```python
from build123d import *

# Parameters (mm, degrees)
CROQUIS1_W                 = 985
CROQUIS1_H                 = 100
SALIENTE_EXTRUIR1_DEPTH    = 12
CROQUIS2_R                 = 18.5
CORTAR_EXTRUIR1_DEPTH      = 1
CORTAR_EXTRUIR1_DEPTH_BACK = 13
CROQUIS3_R                 = 18.5
CORTAR_EXTRUIR2_DEPTH      = 13


with BuildPart() as part:
    # Croquis1 → Saliente-Extruir1 (new body)
    with BuildSketch(Plane.XY):
        with Locations((492.5, 50)):
            Rectangle(CROQUIS1_W, CROQUIS1_H)
    extrude(amount=SALIENTE_EXTRUIR1_DEPTH)

    # Croquis2 → Cortar-Extruir1 (cut, two sides)
    with BuildSketch(Plane.XY.offset(12)) as cortar_extruir1_sk:
        with Locations((74, 36.5)):
            Circle(CROQUIS2_R)
    extrude(amount=CORTAR_EXTRUIR1_DEPTH, mode=Mode.SUBTRACT)
    extrude(cortar_extruir1_sk.sketch, amount=-CORTAR_EXTRUIR1_DEPTH_BACK, mode=Mode.SUBTRACT)

    # Croquis3 → Cortar-Extruir2 (cut, through all)
    with BuildSketch(Plane.XY.offset(12)):
        with Locations((594, 36.5)):
            Circle(CROQUIS3_R)
    extrude(amount=-CORTAR_EXTRUIR2_DEPTH, mode=Mode.SUBTRACT)


solid = part.part
```
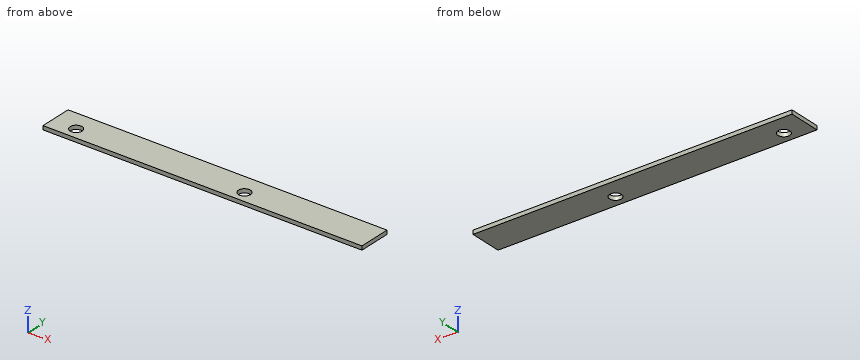
Input: part model. Units: mm. Frame: model coordinates. Give positions to 0.01 mm unless a question says otherwise; leave off trailing zeros. Order: outer loops, then holes, each group sorted by start corner. A loop starts at its lowest first (then second) coordinate and runs counter-clockwise, first axis right, second up. Notation, with made-up numbers: M -34,27.5 L -2,27.5 A13 ccw -2,42.5 Z; hole C 68,-31 d1. An arc over 180 degrees is marked long. Return JSON: item names as keys, results as strings.
Item 1: Cut plane A-A (x = 594). Return loops of the section in (y, z), then the cut area to 3 significant figures.
Solutions:
{"outline": "M 0,0 L 18,0 L 18,12 L 0,12 Z; M 55,0 L 100,0 L 100,12 L 55,12 Z", "area": "756 mm^2"}
Item 2: Ray query, probe 1 along Y at (x, z) = (594, 5.75); probe 2 along X at (y, z) = (47, 7.5). Return the intervals inside material, ascending.
Solutions:
{"probe 1": "0 to 18, 55 to 100", "probe 2": "0 to 58.77, 89.23 to 578.77, 609.23 to 985"}
Item 3: Cut plane C-C (z = 6.5). Return loops of the section in (x, y).
Solutions:
{"outline": "M 0,0 L 985,0 L 985,100 L 0,100 Z; hole C 74,36.5 d37; hole C 594,36.5 d37"}
Item 4: Cut plane B-B (y = 36.5). Return loops of the section in (x, z), then the cut area to 3 significant figures.
Solutions:
{"outline": "M 0,0 L 55.5,0 L 55.5,12 L 0,12 Z; M 92.5,0 L 575.5,0 L 575.5,12 L 92.5,12 Z; M 612.5,0 L 985,0 L 985,12 L 612.5,12 Z", "area": "10,900 mm^2"}
